Geometry: final body of the model. Coordinates: model frame, mm. A direction names the side the tool comes from. Coordinates: 2 decimals unless noted, no trailing zeros. Write each loop counter-clockwise with the first axis right and the second up, starting at its lowest first coordinate (ties: lowest second). Pieces come first, ordered by that corner, then holes. Notation, with made-up numbers: (17.5, 40) - (49.5, 40) arc R27 ccw to (49.5, 58) - close; hole circle Ø5 at (-17, 43.5). An arc over 180 degrees is marked (long way). Put each result on its own line as item: value.
```python
from build123d import *

# Parameters (mm, degrees)
SKETCH1_R           = 5
BOSS_EXTRUDE1_DEPTH = 9.81
SKETCH2_R           = 9
BOSS_EXTRUDE2_DEPTH = 1
SKETCH3_R           = 4
CUT_EXTRUDE1_DEPTH  = 15.72


with BuildPart() as part:
    # Sketch1 → Boss-Extrude1 (new body)
    with BuildSketch(Plane(origin=(0, 0, 0), x_dir=(1, 0, 0), z_dir=(0, 1, 0))):
        Circle(SKETCH1_R)
    extrude(amount=-BOSS_EXTRUDE1_DEPTH)

    # Sketch2 → Boss-Extrude2 (add)
    with BuildSketch(Plane(origin=(0, 0, 0), x_dir=(1, 0, 0), z_dir=(0, 1, 0))):
        Circle(SKETCH2_R)
    extrude(amount=BOSS_EXTRUDE2_DEPTH)

    # Sketch3 → Cut-Extrude1 (cut)
    with BuildSketch(Plane(origin=(0, 1, 0), x_dir=(1, 0, 0), z_dir=(0, 1, 0))):
        Circle(SKETCH3_R)
    extrude(amount=-CUT_EXTRUDE1_DEPTH, mode=Mode.SUBTRACT)


solid = part.part
```
1. Section query C-C (y = 0.5). Return loops of the section in (x, z), then the cut area to 3 significant figures.
Answer below:
outline: circle Ø18 at (0, 0); hole circle Ø8 at (0, 0)
area: 204 mm²
2. Pin query (flat end, axial travel): pin 1 Ø1 at (x, y) = (-2.5, -3.5) entering from -Z; pin 2 Ø4 at (x, y) = (3.5, -1.5) entering from -Z. Return the tip coordinate at first contact, or that it passes through.
Answer below:
pin 1: stops at z = -4.58
pin 2: stops at z = -8.73
3. Section query D-D (z = -6.75). Return loops of the section in (x, y), then the cut area to 3 significant figures.
Answer below:
outline: (-5.95, 0) - (5.95, 0) - (5.95, 1) - (-5.95, 1) - close
area: 11.9 mm²
4. Ray query, probe 1 along X at (y, z) = (-6.25, 0); probe 2 along Y at (x, z) = (7.75, -3.75). Return the intervals inside material, ascending. Write a range as from..to.
Answer below:
probe 1: x = -5..-4, 4..5
probe 2: y = 0..1
5. Section query A-A (z = 0). Return loops of the section in (x, y).
Answer below:
outline: (-9, 0) - (-5, 0) - (-5, -9.81) - (-4, -9.81) - (-4, 1) - (-9, 1) - close; (4, -9.81) - (5, -9.81) - (5, 0) - (9, 0) - (9, 1) - (4, 1) - close
6. Section query B-B (x = 1.5). Return loops of the section in (y, z).
Answer below:
outline: (-9.81, -4.77) - (0, -4.77) - (0, -8.87) - (1, -8.87) - (1, -3.71) - (-9.81, -3.71) - close; (-9.81, 3.71) - (1, 3.71) - (1, 8.87) - (0, 8.87) - (0, 4.77) - (-9.81, 4.77) - close
7. Set-up query: faces 1 (the flat face through (4, 0, 4)), 2 (the cylindrical face through (-1.172, 0.493, -8.923)). Return all of +Z, -Z, +X, -X, +Y, -Y with unobstructed straight access to the full face (end or side cutting, diameter ignored); none if empty.
Answer below:
face 1: -Y
face 2: +Y, -Y
8. Mould query, pull axis Z, two halves, no side actions, for faces 3 (the cylindrical face through (-1.08, -4.84, 4.88)), 4 (the flat face through (4, 1, 2)), 5 (the cylindrical face through (-0.867, -4.329, 3.905)). Classes: +Z half, -Z half, draft (parallel to the pull), parting line (faces both ways), or undercut.
Answer below:
face 3: parting line
face 4: draft
face 5: undercut
